Verification items for the finished model (mm, model axes). Face numbers are marked on the shaded views. A direction names the side the tool comes from. Round coordinates to 2 decimals unless told otherwise and drop trailing zeros. Loops run counter-clockwise (first coordinate to the right, second up) from the corner with the lowest first, then second, coordinate; pieces in that order, holes last. Notation, with made-up numbers: M -30,-38.5 L 25,-38.5 A19 ccw 25,-21.5 Z; hole C 17.25,66.25 d4. An arc over 180 degrees is marked long. One line per item, written item: value.
from build123d import *

# Parameters (mm, degrees)
F0_W     = 86.602568
F0_H     = 152.204066
F1_DEPTH = 5
F2_W     = 10
F2_H     = 2.5
F3_DEPTH = 20


with BuildPart() as f1:
    # F0 (on Top) → F1 (new body)
    with BuildSketch(Plane.XY):
        Rectangle(F0_W, F0_H)
    extrude(amount=F1_DEPTH)

    # F2 (on face) → F3 (join)
    with BuildSketch(Plane(origin=(0, 0, 0), x_dir=(1, 0, 0), z_dir=(0, 0, -1))):
        Polygon((-28.301284, 66.102033), (-33.301284, 66.102033), (-33.301284, 46.102033), (-28.301284, 46.102033), (-28.301284, 48.602033), (-28.301284, 63.602033), align=None)
        with Locations((-23.301284, 64.852033)):
            Rectangle(F2_W, F2_H)
        with Locations((-23.301284, 47.352033)):
            Rectangle(F2_W, F2_H)
        Polygon((28.301284, 48.602033), (28.301284, 46.102033), (33.301284, 46.102033), (33.301284, 66.102033), (28.301284, 66.102033), (28.301284, 63.602033), align=None)
        with Locations((23.301284, 47.352033)):
            Rectangle(F2_W, F2_H)
        with Locations((23.301284, 64.852033)):
            Rectangle(F2_W, F2_H)
    extrude(amount=F3_DEPTH)


solid = f1.part
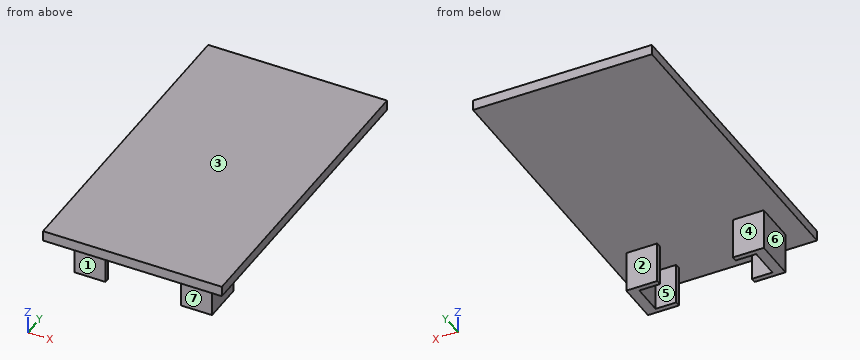
(1) Sectioned sample at C-C on y = -61. Enter the section's corners in (x, z), and give its area (3 significant figures).
Completed:
outline: M -43.3,0 L -33.3,0 L -33.3,-20 L -28.3,-20 L -28.3,0 L 28.3,0 L 28.3,-20 L 33.3,-20 L 33.3,0 L 43.3,0 L 43.3,5 L -43.3,5 Z
area: 633 mm^2
(2) Thickness scan on L1, parallel to Y at x = -19, z = -3.5; L2, parallel to X at y = -54.5, z = -12; L3, parallel to Z at x = -8.5, y = -11. Record the ranges inside material, lowest first. Write a range as from..to.
Completed:
L1: y = -66.1..-63.6, -48.6..-46.1
L2: x = -33.3..-28.3, 28.3..33.3
L3: z = 0..5
(3) Tool access check on the marked faces 1, 2 and 3. Record the directions out of +Z, -Z, +X, -X, +Y, -Y that give a thin tool (end or side, any length) a straight path to the whole face; none if there is none.
Completed:
face 1: -Z, +X, -X, -Y
face 2: -Z, +X, -X, +Y
face 3: +Z, +X, -X, +Y, -Y
(4) Mould release check, pull along Y, two halves, no side actions. Record for the marked faces 4, 5, 6 and 7: +Y half, -Y half, draft (parallel to the pull), parting line (faces both ways), or undercut.
Completed:
face 4: +Y half
face 5: undercut
face 6: draft
face 7: -Y half
(5) Sectioned sample at A-A on z = -8.5. Enter the section's corners in (x, y), and give its area (3 significant figures).
Completed:
outline: M -33.3,-66.1 L -18.3,-66.1 L -18.3,-63.6 L -28.3,-63.6 L -28.3,-48.6 L -18.3,-48.6 L -18.3,-46.1 L -33.3,-46.1 Z; M 18.3,-66.1 L 33.3,-66.1 L 33.3,-46.1 L 18.3,-46.1 L 18.3,-48.6 L 28.3,-48.6 L 28.3,-63.6 L 18.3,-63.6 Z
area: 300 mm^2
(6) Sectioned sample at D-D on x = -1. Enter the section's corners in (y, z).
Completed:
outline: M -76.1,0 L 76.1,0 L 76.1,5 L -76.1,5 Z
(7) Depth check by flat-ended pin: pin 1 Ø5 at (x, z) = (25.5, -14) entering from +Y; pin 2 Ø12 at (x, z) = (-31.5, -9.5) entering from -Y; pin 3 Ø2 at (y, z) = (-64.5, -12.5) entering from +X. Enter the tip coordinate at first touch or a pass-through.
Completed:
pin 1: stops at y = -46.1
pin 2: stops at y = -66.1
pin 3: stops at x = 33.3
(8) Sectioned sample at B-B on x = 30. Enter the section's corners in (y, z), and give its area (3 significant figures).
Completed:
outline: M -76.1,0 L -66.1,0 L -66.1,-20 L -46.1,-20 L -46.1,0 L 76.1,0 L 76.1,5 L -76.1,5 Z
area: 1,160 mm^2
